from build123d import *

# Parameters (mm, degrees)
SKETCH_1_W          = 105
SKETCH_1_H          = 75
SKETCH_1_W_2        = 95
SKETCH_1_H_2        = 65
EXTRUDE_1_DEPTH     = 10
SKETCH_2_W          = 40
SKETCH_2_H          = 40
EXTRUDE_2_DEPTH     = 10
CUT_EXTRUDE_1_REACH = 101.906
SKETCH_3_R          = 7.5
CUT_EXTRUDE_2_REACH = 101.906
SKETCH_4_W          = 70
SKETCH_4_H          = 10
FILLET_2_RADIUS     = 5
FILLET_2_LENGTH     = 40
FILLET_3_SIZE       = 3
SKETCH_8_R          = 1.3
CUT_EXTRUDE_3_DEPTH = 100.906206141
SKETCH_9_W          = 18
SKETCH_9_H          = 50
CUT_EXTRUDE_4_DEPTH = 3


with BuildPart() as part:
    # 草圖1 → 填料-伸長1 (new body)
    with BuildSketch(Plane(origin=(0, 0, 0), x_dir=(1, 0, 0), z_dir=(0, 1, 0))):
        Rectangle(SKETCH_1_W, SKETCH_1_H)
        Rectangle(SKETCH_1_W_2, SKETCH_1_H_2, mode=Mode.SUBTRACT)
    extrude(amount=EXTRUDE_1_DEPTH)

    # 草圖2 → 填料-伸長2 (add)
    with BuildSketch(Plane.XY.offset(37.5)):
        with Locations((0, 20)):
            Rectangle(SKETCH_2_W, SKETCH_2_H)
    extrude(amount=-EXTRUDE_2_DEPTH)

    # 草圖3 → 除料-伸長1 (cut, up to next)
    with BuildSketch(Plane.XY.offset(37.5), mode=Mode.PRIVATE) as cut_extrude_1_sk1:
        with Locations((0, 20)):
            Circle(SKETCH_3_R)
    cut_extrude_1_tool1 = extrude(cut_extrude_1_sk1.sketch, amount=-CUT_EXTRUDE_1_REACH, mode=Mode.PRIVATE) & part.part
    add(cut_extrude_1_tool1.solids().sort_by_distance((0, 20, 37.5))[0], mode=Mode.SUBTRACT)

    # 草圖4 → 除料-伸長2 (cut, up to next)
    with BuildSketch(Plane(origin=(0, 0, -37.5), x_dir=(-1, 0, 0), z_dir=(0, 0, -1)), mode=Mode.PRIVATE) as cut_extrude_2_sk1:
        with Locations((0, 5)):
            Rectangle(SKETCH_4_W, SKETCH_4_H)
    cut_extrude_2_tool1 = extrude(cut_extrude_2_sk1.sketch, amount=-CUT_EXTRUDE_2_REACH, mode=Mode.PRIVATE) & part.part
    add(cut_extrude_2_tool1.solids().sort_by_distance((0, 5, -37.5))[0], mode=Mode.SUBTRACT)

    # 草圖7 → Ø1.0 (1) 直徑孔1 (revolve, cut)
    with BuildSketch(Plane(origin=(20, 32, 32.5), x_dir=(0, 0, -1), z_dir=(0, 1, 0))):
        Polygon((0, 0), (0, 7.881118805), (1.3, 7.1), (1.3, 0), align=None)
    hole_wizard_1_0_1_1 = revolve(axis=Axis((26.35, 32, 32.5), (-1, 0, 0)), mode=Mode.SUBTRACT)

    # 鏡射1: Ø1.0 (1) 直徑孔1 across plane
    add(hole_wizard_1_0_1_1.mirror(Plane(origin=(0, 0, 0), x_dir=(0, 0, 1), z_dir=(1, 0, 0))), mode=Mode.SUBTRACT)

    # 圓角2: full round fillet: the end face becomes a half cylinder, R = half its width
    fillet_2_face = Plane((0, 40, 32.5), x_dir=(1, 0, 0), z_dir=(0, 1, 0))  # on the end face: x along it, z out of the body
    fillet_2_slab = fillet_2_face.offset(-FILLET_2_RADIUS / 2) * Box(FILLET_2_LENGTH, 2 * FILLET_2_RADIUS, FILLET_2_RADIUS, mode=Mode.PRIVATE)  # the body's end, R deep
    fillet_2_round = Plane((0, 35, 32.5), x_dir=(0, 1, 0), z_dir=(1, 0, 0)) * Cylinder(FILLET_2_RADIUS, FILLET_2_LENGTH, mode=Mode.PRIVATE)  # its axis R under the face
    add(fillet_2_slab - fillet_2_round, mode=Mode.SUBTRACT)

    # 圓角3
    # a fillet whose section is not a circle: 3 mm, written as the material it takes off along each edge
    with BuildSketch(Plane(origin=(35, 0, -45), x_dir=(0, 1, 0), z_dir=(0, 0, 1)), Plane(origin=(-35, 10, -45), x_dir=(0, -1, 0), z_dir=(0, 0, 1))) as fillet_3_piece_1:
        with BuildLine():
            Bezier((FILLET_3_SIZE, 0), (0, 0), (0, -FILLET_3_SIZE), weights=[1, 1, 1])
            Line((0, -FILLET_3_SIZE), (0, 0))
            Line((0, 0), (FILLET_3_SIZE, 0))
        make_face()
    extrude(amount=20, mode=Mode.SUBTRACT)
    with BuildSketch(Plane(origin=(35, 10, -45), x_dir=(0, -1, 0), z_dir=(0, 0, 1)), Plane(origin=(-35, 0, -45), x_dir=(0, 1, 0), z_dir=(0, 0, 1))) as fillet_3_piece_2:
        with BuildLine():
            Bezier((FILLET_3_SIZE, 0), (0, 0), (0, FILLET_3_SIZE), weights=[1, 1, 1])
            Line((0, FILLET_3_SIZE), (0, 0))
            Line((0, 0), (FILLET_3_SIZE, 0))
        make_face()
    extrude(amount=20, mode=Mode.SUBTRACT)

    # 草圖8 → 除料-伸長3 (cut, through all)
    with BuildSketch(Plane.XY.offset(37.5)):
        with Locations((-10.5, 32.5)):
            Circle(SKETCH_8_R)
        with Locations((-10.5, 20)):
            Circle(SKETCH_8_R)
        with Locations((10.5, 32.5)):
            Circle(SKETCH_8_R)
        with Locations((10.5, 20)):
            Circle(SKETCH_8_R)
    extrude(amount=-CUT_EXTRUDE_3_DEPTH, mode=Mode.SUBTRACT)

    # 草圖9 → 除料-伸長4 (cut)
    with BuildSketch(Plane.XY.offset(37.5)):
        with Locations((0, 20)):
            Rectangle(SKETCH_9_W, SKETCH_9_H)
    extrude(amount=-CUT_EXTRUDE_4_DEPTH, mode=Mode.SUBTRACT)


solid = part.part
Input: part model. Units: mm. Frame: model coordinates. A direction names the side the tool comes from. Give positions to 0.01 mm unless a question says otherwise; leave off trailing zeros. Write each loop counter-clockwise with the first axis right and the second up, starting at its lowest first coordinate (ties: lowest second). Pieces come first, ordered by that corner, then holes.
Q1. Set-up query: faces 4 (the face through (47.5, 5, 0)), 5 (the face through (-8, 20, 34.5)), 6 (the face through (-35, 5, -35)). Return all of +Z, -Z, +X, -X, +Y, -Y with unobstructed straight access to the full face (end or side cutting, diameter ignored); none if empty.
Q2. Section C-C, the plane z = -28. Output: boundary loops of the cut face in (x, y).
Q3. First-contact query: P1, Ø3, axis at x = 19.5, y = 28.5, coming from the -Z side; P2, Ø5, axis at x = 30.5, y = 5, coming from the -Z side; P3, Ø3, axis at y = 27, z = 33, coming from the -X side. Flat tips, straight axial feed; report the tip coordinate or a pass-through.
Q4. Section A-A, the plane x = 0. Output: boundary loops of the cut face in (y, z), plus the area to 3 significant figures.
Q5. Pull-direction query (X, two-part tool) for faces 1 (the face through (52.5, 5, 1)), 2 (the face through (9, 20, 36)), 3 (the face through (48, 10, 3)); classes: pulls with the +X half, pulls with the -X half, needs draft (parallel to the pull), parting line crosses it, or undercut.
Q6. Material intervals for probe 1 along Y at (x, z) = (-10.5, 32); probe 2 along Y at (x, z) = (-10.5, 34.5); probe 3 along X at (y, z) = (7, 31.5), sorted ascending.
Q7. Section B-B, the plane y = 26. Output: boundary loops of the cut face in (x, z).
Q8. Section D-D, the plane y = 20. Output: boundary loops of the cut face in (x, z).
Filled in:
1. face 4: +Y, -Y
1. face 5: +Z, +Y, -Y
1. face 6: -Z, +Y, -Y
2. outline: (-52.5, 0) - (-47.5, 0) - (-47.5, 10) - (-52.5, 10) - close; (47.5, 0) - (52.5, 0) - (52.5, 10) - (47.5, 10) - close
3. P1: stops at z = 27.5
3. P2: stops at z = 32.5
3. P3: stops at x = -20
4. outline: (0, 27.5) - (12.5, 27.5) - (12.5, 34.5) - (0, 34.5) - close; (27.5, 27.5) - (35, 27.5) arc R5 ccw to (39.58, 34.5) - (27.5, 34.5) - close
4. area: 169 mm2
5. face 1: pulls with the +X half
5. face 2: undercut
5. face 3: needs draft
6. probe 1: y = 0 to 18.7, 21.3 to 31.2, 33.8 to 39.97
6. probe 2: y = 0 to 18.7, 21.3 to 31.2, 33.8 to 39.58
6. probe 3: x = -52.5 to -47.5, -20 to 20, 47.5 to 52.5
7. outline: (-20, 27.5) - (-4.5, 27.5) - (-4.5, 34.5) - (-9, 34.5) - (-9, 37.5) - (-20, 37.5) - close; (4.5, 27.5) - (20, 27.5) - (20, 37.5) - (9, 37.5) - (9, 34.5) - (4.5, 34.5) - close
8. outline: (-20, 27.5) - (-11.8, 27.5) - (-11.8, 37.5) - (-20, 37.5) - close; (-9.2, 27.5) - (-7.5, 27.5) - (-7.5, 34.5) - (-9, 34.5) - (-9, 37.5) - (-9.2, 37.5) - close; (7.5, 27.5) - (9.2, 27.5) - (9.2, 37.5) - (9, 37.5) - (9, 34.5) - (7.5, 34.5) - close; (11.8, 27.5) - (20, 27.5) - (20, 37.5) - (11.8, 37.5) - close
